from build123d import *

# Parameters (mm, degrees)
F0_W           = 3.175
F0_H           = 22.225
F0_H_2         = 3.175
F0_W_2         = 22.225
F1_DEPTH       = 114.3
F3_D           = 4.4958
F3_CSINK_D     = 9.1186
F3_CSINK_ANGLE = 82


with BuildPart() as f1:
    # F0 (on Front) → F1 (new body)
    with BuildSketch(Plane.XZ):
        with Locations((85.725, 14.2875)):
            Rectangle(F0_W, F0_H)
        with Locations((85.725, 1.5875)):
            Rectangle(F0_W, F0_H_2)
        with Locations((73.025, 1.5875)):
            Rectangle(F0_W_2, F0_H_2)
    extrude(amount=F1_DEPTH)

    # F3 (through all)
    with Locations(Plane.XY.offset(3.175)):
        with Locations((73.025, -104.775), (73.025, -9.525)):
            CounterSinkHole(F3_D / 2, F3_CSINK_D / 2, counter_sink_angle=F3_CSINK_ANGLE)


solid = f1.part
Here's how the part is built. I have some questions about the finished solid (model axes, mm). A direction names the side the tool comes from. Round coordinates to 2 decimals unless told otherwise and drop trailing zeros. Order: outer loops, then holes, each group sorted by start corner. A loop starts at its lowest first (then second) coordinate and runs counter-clockwise, first axis right, second up. Notation, with made-up numbers: (8, 12.5) -> (42, 12.5) arc R27 ccw to (42, 36.5) -> close; hole circle Ø2 at (58, 45.25). An arc over 180 degrees is marked (long way). Return JSON: item names as keys, results as strings.
Q1. For pin 1 Ø6 at (x, y) = (68.5, -20) entering from +Z (3 decimals); pin 2 Ø8 at (y, z) = (-32.5, 12.5) entering from -X; pin 3 Ø4 at (x, y) = (76.5, -72.5) entering from -Z, each with a flat end and sliding along its axis, tell me the tip position at first contact or that it passes through.
Filled sheet:
{"pin 1": "stops at z = 3.175", "pin 2": "stops at x = 84.14", "pin 3": "stops at z = 0"}
Q2. Which directions (+Z, -Z, +X, -X, +Y, -Y) give clear straight access to the entire face, cutting with the end or side of a thin tool? Please do faces 1 (the flat face through (80, -114.3, 2)), 2 (the flat face through (84.137, -56, 14)).
Filled sheet:
{"face 1": "+Z, -Z, +X, -X, -Y", "face 2": "+Z, -X, +Y, -Y"}
Q3. If we section it at B-B on y = -77.5: List the corners of the cut face in (x, z) for me (1 decimal).
Filled sheet:
{"outline": "(61.9, 0) -> (87.3, 0) -> (87.3, 25.4) -> (84.1, 25.4) -> (84.1, 3.2) -> (61.9, 3.2) -> close"}
Q4. If we mould it in two halves opening along X, with no side actions, what happens to faces 3 (the flat face through (80, 0, 2)), 4 (the flat face through (87.312, -56, 13)), 5 (the cylindrical face through (74.81, -106.14, 0.25))? For each: released by +X, released by -X, zero draft, split by the parting line, or undercut.
Filled sheet:
{"face 3": "zero draft", "face 4": "released by +X", "face 5": "undercut"}
Q5. If we section it at D-D on z = 2: List the corners of the cut face in (x, y) for me (1 decimal).
Filled sheet:
{"outline": "(61.9, -114.3) -> (87.3, -114.3) -> (87.3, 0) -> (61.9, 0) -> close; hole circle Ø7.1 at (73, -104.8); hole circle Ø7.1 at (73, -9.5)"}
Q6. I need wall thicknesses on line 1 along Z through (x, y) = (69, -41.5) (3 decimals); line 2 along X through (y, z) = (-43, 7.5); line 3 along Z through (x, y) = (69.75, -107). Which ranges of each line are inside material? Lowest first, please. Write a range as from..to.
Filled sheet:
{"line 1": "z = 0..3.175", "line 2": "x = 84.14..87.31", "line 3": "z = 0..2.48"}
Q7. If we section it at C-C on x = 63.5: List the corners of the cut face in (y, z) for me (3 decimals).
Filled sheet:
{"outline": "(-114.3, 0) -> (0, 0) -> (0, 3.175) -> (-114.3, 3.175) -> close"}
Q8. If we section it at A-A on z = 21.25: List the corners of the cut face in (x, y) for me.
Filled sheet:
{"outline": "(84.14, -114.3) -> (87.31, -114.3) -> (87.31, 0) -> (84.14, 0) -> close"}
